```python
from build123d import *

# Parameters (mm, degrees)
F1_DEPTH = 25.4
F2_R     = 6.35
F3_DEPTH = 25.4
F5_DEPTH = 25.4
F7_DEPTH = 25.4


with BuildPart() as f1:
    # F0 (on Front) → F1 (new body)
    with BuildSketch(Plane.XZ):
        Polygon((0, 38.1), (0, 0), (76.2, 0), (76.2, 12.7), (23.4621260909, 12.7), (23.4621260909, 38.1), align=None)
    extrude(amount=F1_DEPTH)

    # F2 (on face) → F3 (cut)
    with BuildSketch(Plane.XZ.offset(25.4)):
        with BuildLine():
            ThreePointArc((11.7310630454, 38.1), (19.7267698627, 34.9655343316), (23.4621260909, 27.2322739337))
            Line((23.4621260909, 27.2322739337), (23.4621260909, 38.1))
            Line((23.4621260909, 38.1), (11.7310630454, 38.1))
        make_face()
        with BuildLine():
            ThreePointArc((0, 27.2322739337), (3.7353562282, 34.9655343316), (11.7310630454, 38.1))
            Line((11.7310630454, 38.1), (0, 38.1))
            Line((0, 38.1), (0, 27.2322739337))
        make_face()
        with Locations((10.7621260909, 25.4370161029)):
            Circle(F2_R)
    extrude(amount=-F3_DEPTH, mode=Mode.SUBTRACT)

    # F4 (on face) → F5 (cut)
    with BuildSketch(Plane.XY.offset(12.7)):
        with BuildLine():
            ThreePointArc((67.9121260909, -12.7), (66.0522541514, -8.2098719395), (61.5621260909, -6.35))
            Line((61.5621260909, -6.35), (61.5621260909, -19.05))
            ThreePointArc((61.5621260909, -19.05), (66.0522541514, -17.1901280605), (67.9121260909, -12.7))
        make_face()
        with BuildLine():
            ThreePointArc((42.5121260909, -12.7), (40.6522541514, -8.2098719395), (36.1621260909, -6.35))
            Line((36.1621260909, -6.35), (36.1621260909, -19.05))
            ThreePointArc((36.1621260909, -19.05), (40.6522541514, -17.1901280605), (42.5121260909, -12.7))
        make_face()
        with BuildLine():
            Line((61.5621260909, -19.05), (61.5621260909, -6.35))
            ThreePointArc((61.5621260909, -6.35), (55.2121260909, -12.7), (61.5621260909, -19.05))
        make_face()
        with BuildLine():
            Line((61.5621260909, -6.35), (36.1621260909, -6.35))
            ThreePointArc((36.1621260909, -6.35), (40.6522541514, -8.2098719395), (42.5121260909, -12.7))
            ThreePointArc((42.5121260909, -12.7), (40.6522541514, -17.1901280605), (36.1621260909, -19.05))
            Line((36.1621260909, -19.05), (61.5621260909, -19.05))
            ThreePointArc((61.5621260909, -19.05), (55.2121260909, -12.7), (61.5621260909, -6.35))
        make_face()
        with BuildLine():
            Line((36.1621260909, -19.05), (36.1621260909, -6.35))
            ThreePointArc((36.1621260909, -6.35), (29.8121260909, -12.7), (36.1621260909, -19.05))
        make_face()
        with BuildLine():
            ThreePointArc((61.5621260909, 0), (74.2621260909, -12.7), (61.5621260909, -25.4))
            Line((61.5621260909, -25.4), (76.2, -25.4))
            Line((76.2, -25.4), (76.2, 0))
            Line((76.2, 0), (61.5621260909, 0))
        make_face()
    extrude(amount=-F5_DEPTH, mode=Mode.SUBTRACT)

    # F6 (on face) → F7 (cut)
    with BuildSketch(Plane.XY.offset(12.7)):
        with BuildLine():
            ThreePointArc((70.4301233526, -3.6088711061), (72.6308384047, -11.4457312958), (72.2394995097, -19.5763141925))
            ThreePointArc((72.2394995097, -19.5763141925), (74.1813649126, -11.2700309235), (70.4301233526, -3.6088711061))
        make_face()
    extrude(amount=-F7_DEPTH, mode=Mode.SUBTRACT)


solid = f1.part
```
Model file for the job. Use its own axes, mm. A direction names the side the tool comes from. Coordinates: 2 decimals unless noted, no trailing zeros. Loops run counter-clockwise (first coordinate to the right, second up) from the corner with the lowest first, then second, coordinate; pieces in that order, holes last. Notation, with made-up numbers: (24.25, 51) -> (72.25, 51) arc R13 cw to (72.25, 74) -> close; hole circle Ø3 at (74, -17). An arc over 180 degrees is marked (long way). Answer as a JSON object with one key per item and string values.
Q1. 3-axis set-ups, long thin cutter, end or side, ignore diameter. For faces 1 (the flat face through (23.462, -13, 20)), 2 (the cylindrical face through (29.814, -12.56, 6.439)), 3 (the cylindrical face through (72.618, -11.332, 6.439)): which of +Z, -Z, +X, -X, +Y, -Y reach the whole face in a straight line?
Report:
{"face 1": "+Z, +X, +Y, -Y", "face 2": "+Z, -Z", "face 3": "+Z, -Z, +X"}
Q2. Cut at D-D (y = -21). List the corners of the cut face in (x, z), and give its area (3 significant figures).
Report:
{"outline": "(0, 0) -> (71.17, 0) -> (71.17, 12.7) -> (23.46, 12.7) -> (23.46, 27.23) arc R11.77 ccw to (0, 27.23) -> close; hole circle Ø12.7 at (10.76, 25.44)", "area": "1,310 mm2"}
Q3. Cut at C-C (z = 28). List the corners of the cut face in (x, y).
Report:
{"outline": "(0.08, -25.4) -> (4.95, -25.4) -> (4.95, 0) -> (0.08, 0) -> close; (16.57, -25.4) -> (23.38, -25.4) -> (23.38, 0) -> (16.57, 0) -> close"}
Q4. Cut at A-A (y = -11.5). List the corners of the cut face in (x, z).
Report:
{"outline": "(0, 0) -> (29.93, 0) -> (29.93, 12.7) -> (23.46, 12.7) -> (23.46, 27.23) arc R11.77 ccw to (0, 27.23) -> close; (67.8, 0) -> (72.64, 0) -> (72.64, 12.7) -> (67.8, 12.7) -> close; hole circle Ø12.7 at (10.76, 25.44)"}
Q5. Flat gauge pins, fed straight in: P1, Ø1.5, axis at x = 38.5, y = -20.5, coming from the +Z side; P2, Ø8, axis at x = 27.5, z = 22, coming from the +Y side; P3, Ø8, axis at y = -4, z = 26.5, coming from the +X side. Where does each tip first touch, or does it go through?
Report:
{"P1": "stops at z = 12.7", "P2": "passes through", "P3": "stops at x = 23.46"}
Q6. Cut at B-B (x = 42). List the corners of the cut face in (y, z).
Report:
{"outline": "(-25.4, 0) -> (-19.05, 0) -> (-19.05, 12.7) -> (-25.4, 12.7) -> close; (-6.35, 0) -> (0, 0) -> (0, 12.7) -> (-6.35, 12.7) -> close"}
Q7. Pull direction Y, two halves, no side cores. Call faces 4 (the flat face through (49, -19.05, 6)), 5 (the flat face through (24, 0, 11)), 6 (the cylindrical face through (9.386, -12.878, 19.238)): released by +Y, released by -Y, zero draft, split by the parting line, or undercut.
Report:
{"face 4": "undercut", "face 5": "released by +Y", "face 6": "zero draft"}
Q8. Probe probe 1 along X at (y, z) = (-13, 25); probe 2 along Z at (x, y) = (36, -4.5); probe 3 along X at (y, z) = (-15.75, 4). List the from-to ranges inside material, lowest first.
Report:
{"probe 1": "x = 0 to 4.43, 17.1 to 23.46", "probe 2": "z = 0 to 12.7", "probe 3": "x = 0 to 30.59, 67.13 to 72.75"}
